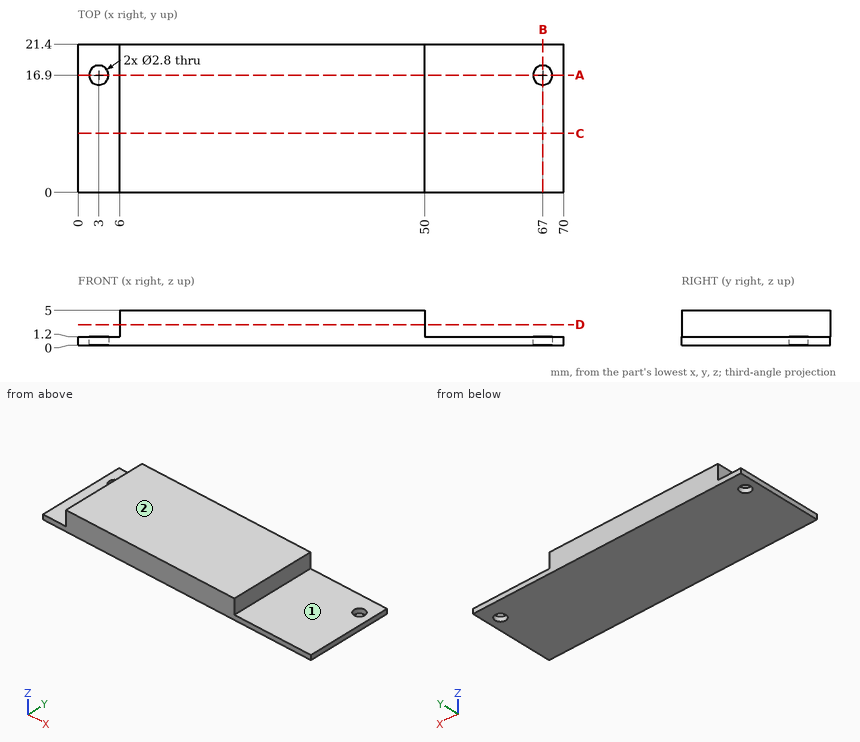
Job drawing, mm, ordinate dimensions from the low corner. One solid piece. A direction names the side the tool comes from. Give positions to 0.01 mm unless a question says otherwise; leave off trailing zeros. Loops run counter-clockwise (first coordinate to the right, second up) from the corner with the lowest first, then second, coordinate; pieces in that order, holes last. Notation, with made-up numbers: M 11.25,47 L 48.25,47 A4 cw 48.25,54 Z; hole C 68.25,19 d5. An arc over 180 degrees is marked long. Put each result on its own line as item: value. Start each with the question number.
1) Saw through at B-B (x = 67). List the corners of the cut face in (y, z).
2) Probe probe 1 along X at (y, z) = (16, 1.05); probe 2 along Y at (x, z) = (67, 0.6); probe 3 along X at (y, z) = (18, 0.6). List the from-to ranges inside material, lowest first.
3) 3-axis set-ups, long thin cutter, end or side, ignore diameter. For the marked faces 1 and 2: which of +Z, -Z, +X, -X, +Y, -Y reach the whole face in a straight line?
4) Flat gauge pins, fed straight in: pin 1 (1.5 mm diameter, centred on y = 13, z = 1, fed in from -X); pin 2 (1.5 mm diameter, centred on y = 12, z = 2.5, fed in from +X). Where does each tip first touch, or does it go through?
5) Saw through at C-C (y = 8.5). List the corners of the cut face in (x, z).
6) Saw through at D-D (z = 2.95). List the corners of the cut face in (x, y), then the cut area to 3 significant figures.
7) Saw through at A-A (y = 16.9). List the corners of the cut face in (x, z), then the cut area to 3 significant figures.
Numbers:
1. outline: M 0,0 L 15.5,0 L 15.5,1.2 L 0,1.2 Z; M 18.3,0 L 21.4,0 L 21.4,1.2 L 18.3,1.2 Z
2. probe 1: 0 to 1.93, 4.07 to 65.93, 68.07 to 70
2. probe 2: 0 to 15.5, 18.3 to 21.4
2. probe 3: 0 to 2.13, 3.87 to 66.13, 67.87 to 70
3. face 1: +Z, +X, +Y, -Y
3. face 2: +Z, +X, -X, +Y, -Y
4. pin 1: x = 0
4. pin 2: x = 50
5. outline: M 0,0 L 70,0 L 70,1.2 L 50,1.2 L 50,5 L 6,5 L 6,1.2 L 0,1.2 Z
6. outline: M 6,0 L 50,0 L 50,21.4 L 6,21.4 Z
6. area: 942 mm^2
7. outline: M 0,0 L 1.6,0 L 1.6,1.2 L 0,1.2 Z; M 4.4,0 L 65.6,0 L 65.6,1.2 L 50,1.2 L 50,5 L 6,5 L 6,1.2 L 4.4,1.2 Z; M 68.4,0 L 70,0 L 70,1.2 L 68.4,1.2 Z
7. area: 244 mm^2
